```python
from build123d import *

# Parameters (mm, degrees)
BOSS_EXTRUDE1_DEPTH      = 152.4
BOSS_EXTRUDE1_DEPTH_BACK = 152.4
SKETCH3_W                = 25.4
SKETCH3_H                = 25.4
SKETCH3_W_2              = 19.05
SKETCH3_H_2              = 19.05
SKETCH6_R                = 3.175
CUT_EXTRUDE1_DEPTH       = 156.02325632


with BuildPart() as part:
    # Sketch3 → Boss-Extrude1 (new, two sides: drawn at the far end of the back side and taken through both)
    with BuildSketch(Plane.XY.offset(-BOSS_EXTRUDE1_DEPTH_BACK)):
        Rectangle(SKETCH3_W, SKETCH3_H)
        Rectangle(SKETCH3_W_2, SKETCH3_H_2, mode=Mode.SUBTRACT)
    extrude(amount=BOSS_EXTRUDE1_DEPTH + BOSS_EXTRUDE1_DEPTH_BACK)

    # Sketch6 → Cut-Extrude1 (cut, through all)
    with BuildSketch(Plane(origin=(0, 12.7, 0), x_dir=(1, 0, 0), z_dir=(0, 1, 0))):
        with Locations(Location((0, -95.25, 0), (0, 0, 270))):
            Circle(SKETCH6_R)
        with Locations(Location((0, 95.25, 0), (0, 0, 90))):
            Circle(SKETCH6_R)
    extrude(amount=-CUT_EXTRUDE1_DEPTH, mode=Mode.SUBTRACT)


solid = part.part
```
Model file for the job. Use its own axes, mm. A direction names the side the tool comes from. Give positions to 0.01 mm unless a question says otherwise; leave off trailing zeros. Order: outer loops, then holes, each group sorted by start corner. A loop starts at its lowest first (then second) coordinate and runs counter-clockwise, first axis right, second up.
1) Wall check: probe 1 along X at (y, z) = (11.95, -95.25) (3 decimals); probe 2 along X at (y, z) = (-2, 123) (3 decimals). Give the ranges that are in metal, low to high.
2) Saw through at A-A, the plane x = 0. Write the cut outline in (y, z) (3 decimals).
3) Saw through at D-D, the plane z = 95.25. Write the cut outline in (x, y) (3 decimals).
4) Saw through at C-C, the plane y = 3.5. Write the cut outline in (x, z) (3 decimals), then the cut area to 3 significant figures.
5) Saw through at B-B, the plane z = -27.5. Write the cut outline in (x, y) (3 decimals).
6) Pin check, flat tip, straight feed: pin 1 (5 mm diameter, centred on x = 0, z = -95.25, fed in from +Y). Stop position of the tip, or through.
7) 3-axis set-ups, long thin cutter, end or side, ignore diameter. For faces 1 (the flat face through (0, -9.525, -2)), 2 (the flat face through (0, -12.7, -2)): which of +Z, -Z, +X, -X, +Y, -Y reach the whole face in a straight line?
8) Mould opens along Z. For faces 3 (the cylindrical face through (0.95, -11.09, 98.28)), 4 (the cylindrical face through (-0.95, -11.09, -98.28)), 5 (the flat face through (9.525, 0, -2)), 6 (the flat face through (11, 0, -152.4)) say: +Z half, -Z half, draft (parallel to the pull), parting line (faces both ways), or undercut.
Computed:
1. probe 1: x = -12.7 to -3.175, 3.175 to 12.7
1. probe 2: x = -12.7 to -9.525, 9.525 to 12.7
2. outline: (-12.7, -152.4) - (-9.525, -152.4) - (-9.525, -98.425) - (-12.7, -98.425) - close; (-12.7, -92.075) - (-9.525, -92.075) - (-9.525, 92.075) - (-12.7, 92.075) - close; (-12.7, 98.425) - (-9.525, 98.425) - (-9.525, 152.4) - (-12.7, 152.4) - close; (9.525, -152.4) - (12.7, -152.4) - (12.7, -98.425) - (9.525, -98.425) - close; (9.525, -92.075) - (12.7, -92.075) - (12.7, 92.075) - (9.525, 92.075) - close; (9.525, 98.425) - (12.7, 98.425) - (12.7, 152.4) - (9.525, 152.4) - close
3. outline: (-12.7, -12.7) - (-3.175, -12.7) - (-3.175, -9.525) - (-9.525, -9.525) - (-9.525, 9.525) - (-3.175, 9.525) - (-3.175, 12.7) - (-12.7, 12.7) - close; (3.175, -12.7) - (12.7, -12.7) - (12.7, 12.7) - (3.175, 12.7) - (3.175, 9.525) - (9.525, 9.525) - (9.525, -9.525) - (3.175, -9.525) - close
4. outline: (-12.7, -152.4) - (-9.525, -152.4) - (-9.525, 152.4) - (-12.7, 152.4) - close; (9.525, -152.4) - (12.7, -152.4) - (12.7, 152.4) - (9.525, 152.4) - close
4. area: 1,940 mm2
5. outline: (-12.7, -12.7) - (12.7, -12.7) - (12.7, 12.7) - (-12.7, 12.7) - close; hole (-9.525, -9.525) - (9.525, -9.525) - (9.525, 9.525) - (-9.525, 9.525) - close
6. pin 1: passes through
7. face 1: +Z, -Z
7. face 2: +Z, -Z, +X, -X, -Y
8. face 3: undercut
8. face 4: undercut
8. face 5: draft
8. face 6: -Z half
